Read the model definition and answer for the solid it produces. Units are mm, in the model's axes. A direction names the side the tool comes from. Coordinates: 2 decimals unless noted, no trailing zeros. Order: outer loops, then holes, each group sorted by start corner. A loop starts at its lowest first (then second) coordinate and runs counter-clockwise, first axis right, second up. Notation, with made-up numbers: (72.5, 18) -> (113.5, 18) arc R12 cw to (113.5, 41) -> close; hole circle Ø8 at (75.25, -18). An arc over 180 degrees is marked (long way). Return JSON: item names as keys, results as strings. Group by question number.
```python
from build123d import *

# Parameters (mm, degrees)
BOSS_EXTRUDE1_DEPTH = 30
BOSS_EXTRUDE3_DEPTH = 4


with BuildPart() as part:
    # Sketch1 → Boss-Extrude1 (new body)
    with BuildSketch(Plane.XY):
        Polygon((7.95, 0), (7.95, -2.04), (4.048, -6.152414984), (-4.048, -6.152414984), (-7.95, -2.04), (-7.95, 0), align=None)
    extrude(amount=BOSS_EXTRUDE1_DEPTH)

    # Sketch2 → Boss-Extrude3 (add, symmetric)
    with BuildSketch(Plane.ZY):
        Polygon((0, 0), (10.751038486, 28.007412795), (10.751038486, 0), align=None)
    extrude(amount=BOSS_EXTRUDE3_DEPTH, both=True)


solid = part.part
```
1. Find section C-C on y = -2.5. Determine the outline of the cut face in (x, z).
2. Given pin 1 (10 mm diameter, centred on y = 13.5, z = 5, fed in from -X); pin 2 (4 mm diameter, centred on x = 0.5, y = 8.5, fed in from +Z); pin 3 (4 mm diameter, centred on y = 17, z = 10, fed in from +X); pin 4 (6 mm diameter, centred on x = 5, z = 23.5, fed in from -Y), each flat-ended and moving along its own axis, determine where each tip first touches the part or whether it passes through.
3. Which of the six approach directions +Z, -Z, +X, -X, +Y, -Y give full straight-line access (tool end or side, diameter ignored) to faces 1 (the face through (0, 14, 10.751)), 2 (the face through (-4, 8, 8)), 3 (the face through (4, 8, 8)), 4 (the face through (0, -3, 30))?
4. Find section D-D on z = 3. Determine the outline of the cut face in (x, y), and give its area (3 significant figures).
5. Find section B-B on z = 28. Determine the outline of the cut face in (x, y), and give its area (3 significant figures).
6. Find section A-A on x = 3. Determine the outline of the cut face in (y, z), and give its area (3 significant figures).
7. Straight lines are drawn through the part: L1, parallel to Y at x = -1, z = 24.75; L2, parallel to X at y = 11.5, z = 5; L3, parallel to Y at x = 5, z = 13.5. For each, find the intervals that lie inside material, in ascending order.
Result:
{
 "1": {"outline": "(-7.51, 0) -> (7.51, 0) -> (7.51, 30) -> (-7.51, 30) -> close"},
 "2": {"pin 1": "x = -4", "pin 2": "z = 10.75", "pin 3": "x = 4", "pin 4": "y = -6.15"},
 "3": {"face 1": "+Z, +X, -X, +Y", "face 2": "+Z, -Z, -X, +Y", "face 3": "+Z, -Z, +X, +Y", "face 4": "+Z, +X, -X, +Y, -Y"},
 "4": {"outline": "(-7.95, -2.04) -> (-4.05, -6.15) -> (4.05, -6.15) -> (7.95, -2.04) -> (7.95, 0) -> (4, 0) -> (4, 7.82) -> (-4, 7.82) -> (-4, 0) -> (-7.95, 0) -> close", "area": "144 mm^2"},
 "5": {"outline": "(-7.95, -2.04) -> (-4.05, -6.15) -> (4.05, -6.15) -> (7.95, -2.04) -> (7.95, 0) -> (-7.95, 0) -> close", "area": "81.8 mm^2"},
 "6": {"outline": "(-6.15, 0) -> (0, 0) -> (28.01, 10.75) -> (0, 10.75) -> (0, 30) -> (-6.15, 30) -> close", "area": "335 mm^2"},
 "7": {"L1": "-6.15 to 0", "L2": "-4 to 4", "L3": "-5.15 to 0"}
}
